from build123d import *

# Parameters (mm, degrees)
BOSS_EXTRUDE4_DEPTH = 15
BOSS_EXTRUDE5_DEPTH = 15
SKETCH3_R           = 8
CUT_EXTRUDE2_DEPTH  = 15
CUT_EXTRUDE3_DEPTH  = 5
SKETCH5_W           = 23.42124253
SKETCH5_H           = 18.287225632
CUT_EXTRUDE5_DEPTH  = 3
SKETCH6_W           = 19.984458363
SKETCH6_H           = 20.131216134
CUT_EXTRUDE7_DEPTH  = 2
SKETCH7_W           = 16.913194531
SKETCH7_H           = 80.268822813
CUT_EXTRUDE8_DEPTH  = 3
SKETCH8_W           = 15.481131963
SKETCH8_H           = 83.563031186
CUT_EXTRUDE9_DEPTH  = 3


with BuildPart() as part:
    # Sketch1 → Boss-Extrude4 (new body)
    with BuildSketch(Plane.XY):
        with BuildLine():
            Line((-15, 120), (15, 120))
            ThreePointArc((15, 120), (22.071067812, 117.071067812), (25, 110))
            Line((25, 110), (25, 10))
            ThreePointArc((25, 10), (22.071067812, 2.928932188), (15, 0))
            Line((15, 0), (-15, 0))
            ThreePointArc((-15, 0), (-22.071067812, 2.928932188), (-25, 10))
            Line((-25, 10), (-25, 110))
            ThreePointArc((-25, 110), (-22.071067812, 117.071067812), (-15, 120))
        make_face()
    extrude(amount=BOSS_EXTRUDE4_DEPTH)

    # Sketch2 → Boss-Extrude5 (add)
    with BuildSketch(Plane.XY.offset(15)):
        with BuildLine():
            Line((15, 120), (0, 120))
            Line((0, 120), (0, 0))
            Line((0, 0), (15, 0))
            ThreePointArc((15, 0), (22.071067812, 2.928932188), (25, 10))
            Line((25, 10), (25, 110))
            ThreePointArc((25, 110), (22.071067812, 117.071067812), (15, 120))
        make_face()
        with BuildLine():
            Line((0, 0), (0, 120))
            Line((0, 120), (-15, 120))
            ThreePointArc((-15, 120), (-22.071067812, 117.071067812), (-25, 110))
            Line((-25, 110), (-25, 10))
            ThreePointArc((-25, 10), (-22.071067812, 2.928932188), (-15, 0))
            Line((-15, 0), (0, 0))
        make_face()
    extrude(amount=BOSS_EXTRUDE5_DEPTH)

    # Sketch3 → Cut-Extrude2 (cut)
    with BuildSketch(Plane.XY.offset(30)):
        with Locations((-12.033216968, 109.656218371)):
            Circle(SKETCH3_R)
        with Locations((-12.033216968, 90.176581151)):
            Circle(SKETCH3_R)
        with Locations((-12.033216968, 70.997837903)):
            Circle(SKETCH3_R)
        with Locations((-12.033216968, 50.457885697)):
            Circle(SKETCH3_R)
        with Locations((-12.033216968, 31.422403349)):
            Circle(SKETCH3_R)
        with Locations((-12.033216968, 12.050211805)):
            Circle(SKETCH3_R)
        with Locations(Location((12.033216968, 12.050211805, 0), (0, 0, 180))):
            Circle(SKETCH3_R)
        with Locations(Location((12.033216968, 31.422403349, 0), (0, 0, 180))):
            Circle(SKETCH3_R)
        with Locations(Location((12.033216968, 50.457885697, 0), (0, 0, 180))):
            Circle(SKETCH3_R)
        with Locations(Location((12.033216968, 70.997837903, 0), (0, 0, 180))):
            Circle(SKETCH3_R)
        with Locations(Location((12.033216968, 90.176581151, 0), (0, 0, 180))):
            Circle(SKETCH3_R)
        with Locations(Location((12.033216968, 109.656218371, 0), (0, 0, 180))):
            Circle(SKETCH3_R)
    extrude(amount=-CUT_EXTRUDE2_DEPTH, mode=Mode.SUBTRACT)

    # Sketch4 → Cut-Extrude3 (cut)
    with BuildSketch(Plane.XY.offset(30)):
        with BuildLine():
            Line((-1.612294676, 13.790891011), (-1.612294676, 102.589988378))
            ThreePointArc((-1.612294676, 102.589988378), (0, 104.202283053), (1.612294676, 102.589988378))
            Line((1.612294676, 102.589988378), (1.612294676, 13.790891011))
            ThreePointArc((1.612294676, 13.790891011), (0, 12.178596336), (-1.612294676, 13.790891011))
        make_face()
    extrude(amount=-CUT_EXTRUDE3_DEPTH, mode=Mode.SUBTRACT)

    # Sketch5 → Cut-Extrude5 (cut)
    with BuildSketch(Plane(origin=(0, 0, 0), x_dir=(-1, 0, 0), z_dir=(0, -1, 0))):
        with Locations((1.812031263, -14.475485378)):
            Rectangle(SKETCH5_W, SKETCH5_H)
    extrude(amount=-CUT_EXTRUDE5_DEPTH, mode=Mode.SUBTRACT)

    # Sketch6 → Cut-Extrude7 (cut)
    with BuildSketch(Plane(origin=(0, 120, 0), x_dir=(1, 0, 0), z_dir=(0, 1, 0))):
        with Locations((-1.103321986, -15.673777661)):
            Rectangle(SKETCH6_W, SKETCH6_H)
    extrude(amount=-CUT_EXTRUDE7_DEPTH, mode=Mode.SUBTRACT)

    # Sketch7 → Cut-Extrude8 (cut)
    with BuildSketch(Plane.ZY.offset(25)):
        with Locations((14.78025647, 58.832283621)):
            Rectangle(SKETCH7_W, SKETCH7_H)
    extrude(amount=-CUT_EXTRUDE8_DEPTH, mode=Mode.SUBTRACT)

    # Sketch8 → Cut-Extrude9 (cut)
    with BuildSketch(Plane(origin=(25, 0, 0), x_dir=(0, 0, -1), z_dir=(1, 0, 0))):
        with Locations((-13.31664767, 60.895190622)):
            Rectangle(SKETCH8_W, SKETCH8_H)
    extrude(amount=-CUT_EXTRUDE9_DEPTH, mode=Mode.SUBTRACT)


solid = part.part
Read the model definition and answer for the solid it produces. Units are mm, in the model's axes. A direction names the side the tool comes from. Round coordinates to 2 decimals unless told otherwise and drop trailing zeros. Loops run counter-clockwise (first coordinate to the right, second up) from the corner with the lowest first, then second, coordinate; pieces in that order, holes last. Notation, with made-up numbers: (-8, 67.25) - (43, 67.25) arc R31 ccw to (43, 96.25) - close; hole circle Ø4 at (69.5, -19). An arc over 180 degrees is marked (long way). One line per question, with ' | ' between items. Start each with the question number.
Q1. Section A-A on z = 27 is taken. Count the separate pieces of the cut face and the enclosed holes in it, plus the area to 3 significant figures.
Q2. Flat-ended cylindrical pins translate along their axes: pin 1 (0.6 mm diameter, centred on y = 118.5, z = 17.5, fed in from +X); pin 2 (1.5 mm diameter, centred on x = 0, z = 8, fed in from +Y); pin 3 (13 mm diameter, centred on x = 13, y = 32.5, fed in from +Z). Find the tip coordinate at first contact, or state that the pin passes through.
Q3. For a pull along Y with two mould halves and no side action, classify faces 4 (the cylindrical face through (13.075, 63.066, 22.605)), 5 (the flat face through (0, 0, 5)), 6 (the flat face through (10, 120, 15)) as +Y half, -Y half, draft (parallel to the pull), parting line (faces both ways), or undercut.
Q4. Section C-C on z = 8.75 is taken. Give the vertices of the cut face in (x, y), plus the area to 3 significant figures.
Q5. Find the intervals of material crossed by L1, parallel to X at y = 14.5, z = 22.75; L2, parallel to Z at x = -22.5, y = 50.5; L3, parallel to X at y = 55, z = 16.5, in increasing order.
Q6. Section B-B on x = 0 is taken. Give the vertices of the cut face in (y, z).
Q7. For faces 1 (the cylindrical face through (-13.07, 117.59, 22.6)), 2 (the flat face through (-24, 58, 23.237)), 3 (the flat face through (-13.523, 1, 15)), determine the directions among +Z, -Z, +X, -X, +Y, -Y from which every point of the face is accessible in a straight line to the end or side of a thin tool.
Established:
1) separate pieces: 1 | enclosed holes: 13 | area: 3,210 mm²
2) pin 1: x = 20.72 | pin 2: y = 118 | pin 3: z = 15
3) face 4: undercut | face 5: -Y half | face 6: +Y half
4) outline: (-25, 10) arc R10 ccw to (-15, 0) - (-13.52, 0) - (-13.52, 3) - (9.9, 3) - (9.9, 0) - (15, 0) arc R10 ccw to (25, 10) - (25, 19.11) - (22, 19.11) - (22, 102.68) - (25, 102.68) - (25, 110) arc R10 ccw to (15, 120) - (8.89, 120) - (8.89, 118) - (-11.1, 118) - (-11.1, 120) - (-15, 120) arc R10 ccw to (-25, 110) - (-25, 98.97) - (-22, 98.97) - (-22, 18.7) - (-25, 18.7) - close | area: 5,310 mm²
5) L1: -25 to -19.65, -4.42 to 4.42, 19.65 to 25 | L2: 0 to 6.32, 23.24 to 30 | L3: -22 to -18.62, -5.45 to 5.45, 18.62 to 22
6) outline: (0, 0) - (120, 0) - (120, 5.61) - (118, 5.61) - (118, 25.74) - (120, 25.74) - (120, 30) - (104.2, 30) - (104.2, 25) - (12.18, 25) - (12.18, 30) - (0, 30) - (0, 23.62) - (3, 23.62) - (3, 5.33) - (0, 5.33) - close
7) face 1: +Z | face 2: -X | face 3: -Y
